CAD build for the part. Positions are in the model's coordinates, mm. Face numbers are marked on the shaded views. A direction names the side the tool comes from. Coordinates: 2 decimals unless noted, no trailing zeros. Loops run counter-clockwise (first coordinate to the right, second up) from the corner with the lowest first, then second, coordinate; pieces in that order, holes last. Notation, with made-up numbers: (-2.75, 81.25) -> (51.25, 81.25) arc R16 ccw to (51.25, 95.25) -> close; hole circle Ø3 at (-15.5, -4). An arc over 180 degrees is marked (long way). Write each question's results on one line, items separated by ' | '.
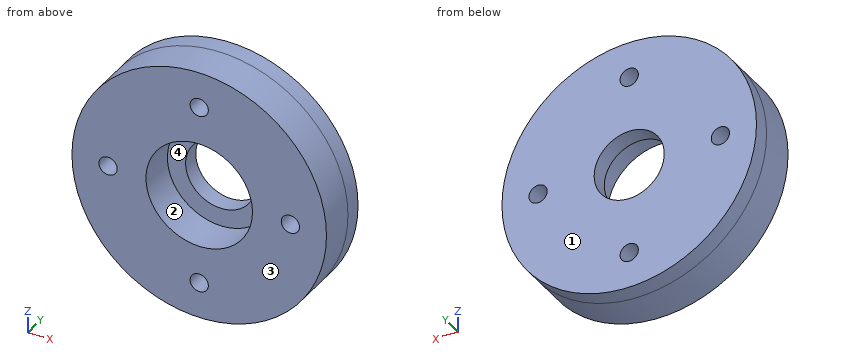
```python
from build123d import *

# Parameters (mm, degrees)
SKETCH_1_R               = 18.15
SKETCH_1_R_2             = 7.6
EXTRUDE_1_DEPTH          = 5.3
SKETCH_8_R               = 18.15
SKETCH_8_R_2             = 5
EXTRUDE_6_DEPTH          = 2.5
SKETCH_9_R               = 1.3
CUT_EXTRUDE_3_DEPTH      = 8.8
PATTERN_CIRCULAR_1_COUNT = 4


with BuildPart() as part:
    # Эскиз1 → Бобышка-Вытянуть1 (new body)
    with BuildSketch(Plane(origin=(0, 0, 0), x_dir=(1, 0, 0), z_dir=(0, 1, 0))):
        Circle(SKETCH_1_R)
        Circle(SKETCH_1_R_2, mode=Mode.SUBTRACT)
    extrude(amount=EXTRUDE_1_DEPTH)

    # Эскиз8 → Бобышка-Вытянуть6 (add)
    with BuildSketch(Plane.XZ.offset(-5.3)):
        Circle(SKETCH_8_R)
        Circle(SKETCH_8_R_2, mode=Mode.SUBTRACT)
    extrude(amount=-EXTRUDE_6_DEPTH)

    # Эскиз9 → Вырез-Вытянуть3 (cut, through all)
    with BuildSketch(Plane(origin=(0, 7.8, 0), x_dir=(1, 0, 0), z_dir=(0, 1, 0))):
        with Locations((0, 13)):
            Circle(SKETCH_9_R)
    cut_extrude_3 = extrude(amount=-CUT_EXTRUDE_3_DEPTH, mode=Mode.SUBTRACT)

    # Круговой массив1: Вырез-Вытянуть3 ×4 about axis
    pattern_circular_1_axis = Axis((0, 0, 0), (0, 1, 0))
    for i in range(1, PATTERN_CIRCULAR_1_COUNT):
        add(cut_extrude_3.rotate(pattern_circular_1_axis, i * 360 / PATTERN_CIRCULAR_1_COUNT), mode=Mode.SUBTRACT)


solid = part.part
```
Q1. Which spindle directions (+Z, -Z, +X, -X, +Y, -Y) get a long thin tool onto all of the face, cutting with end or side? Do the marked faces 1 and 2. Say none if no direction does.
Results are:
face 1: +Z, -Z, +X, -X, +Y | face 2: -Y
Q2. Cut at D-D on x = -13.5. Write the cut outline in (y, z).
Results are:
outline: (0, -12.13) -> (7.8, -12.13) -> (7.8, -1.2) -> (0, -1.2) -> close; (0, 1.2) -> (7.8, 1.2) -> (7.8, 12.13) -> (0, 12.13) -> close
Q3. Pull direction Z, two halves, no side cores. Call the marked faces 3 and 4: +Z half, -Z half, draft (parallel to the pull), parting line (faces both ways), or undercut.
Results are:
face 3: draft | face 4: undercut
Q4. Cut at B-B on y = 1. Write the cut outline in (x, z), and give its area (3 significant figures).
Results are:
outline: circle Ø36.3 at (0, 0); hole circle Ø2.6 at (-13, 0); hole circle Ø15.2 at (0, 0); hole circle Ø2.6 at (0, -13); hole circle Ø2.6 at (0, 13); hole circle Ø2.6 at (13, 0) | area: 832 mm^2
Q5. Wall check: L1, parallel to Z at x = 0, y = 6; L2, parallel to Z at x = 0, y = 4.5. Give the ranges that are in metal, low to high. Write a range as from..to.
Results are:
L1: -18.15..-14.3, -11.7..-5, 5..11.7, 14.3..18.15 | L2: -18.15..-14.3, -11.7..-7.6, 7.6..11.7, 14.3..18.15
Q6. Cut at A-A on x = 0. Write the cut outline in (y, z), and give its area (3 significant figures).
Results are:
outline: (0, -18.15) -> (7.8, -18.15) -> (7.8, -14.3) -> (0, -14.3) -> close; (0, -11.7) -> (7.8, -11.7) -> (7.8, -5) -> (5.3, -5) -> (5.3, -7.6) -> (0, -7.6) -> close; (0, 7.6) -> (5.3, 7.6) -> (5.3, 5) -> (7.8, 5) -> (7.8, 11.7) -> (0, 11.7) -> close; (0, 14.3) -> (7.8, 14.3) -> (7.8, 18.15) -> (0, 18.15) -> close | area: 137 mm^2
Q7. Cut at C-C on z = 0. Write the cut outline in (x, y), and give its area (3 significant figures).
Results are:
outline: (-18.15, 0) -> (-14.3, 0) -> (-14.3, 7.8) -> (-18.15, 7.8) -> close; (-11.7, 0) -> (-7.6, 0) -> (-7.6, 5.3) -> (-5, 5.3) -> (-5, 7.8) -> (-11.7, 7.8) -> close; (5, 5.3) -> (7.6, 5.3) -> (7.6, 0) -> (11.7, 0) -> (11.7, 7.8) -> (5, 7.8) -> close; (14.3, 0) -> (18.15, 0) -> (18.15, 7.8) -> (14.3, 7.8) -> close | area: 137 mm^2
Q8. Drop flat-ended pins along their axis: pin 1 (1 mm diameter, centred on y = 3, z = -11.5, fed in from -X); pin 2 (4 mm diameter, centred on y = 1, z = -9.5, fed in from -X); pin 3 (12 mm diameter, centred on x = 0, z = 0, fed in from -Y). Give the stop position or say it passes through.
Results are:
pin 1: x = -14.44 | pin 2: x = -16.53 | pin 3: y = 5.3
